Here's how the part is built. I have some questions about the finished solid (model axes, mm). A direction names the side the tool comes from. Round coordinates to 2 decimals unless told otherwise and drop trailing zeros. Write each loop counter-clockwise with the first axis right and the second up, starting at its lowest first coordinate (ties: lowest second). Pieces come first, ordered by that corner, then holes. Notation, with made-up numbers: (31, -24.75) - (66, -24.75) arc R21 ccw to (66, -20.75) - close; hole circle Ø9 at (44.5, 87). An arc over 180 degrees is marked (long way). Use one line per item in the form item = value. Start each with the question number.
1. I want a section at A-A, the plane x = 60. List the corners of the cut face in (y, z) for me.
2. I want a section at C-C, the plane y = 6. List the corners of the cut face in (x, z) for me.
3. I want a section at D-D, the plane x = 35. List the corners of the cut face in (y, z) for me.
4. I want a section at B-B, the plane z = 2. List the corners of the cut face in (x, y) for me.
5. Will these pins go through, and if not, where does the flat tip stop? pin 1 (6.5 mm diameter, centred on x = 6, y = 10, fed in from -Z); pin 2 (10 mm diameter, centred on x = 33, y = 7, fed in from -Z); pin 3 (1.5 mm diameter, centred on y = 3.5, z = 3.5, fed in from +X); pin 4 (2 mm diameter, centred on x = 62.5, z = 3.5, fed in from -Y).
6. If I drill on line 1 along X through (y, z) = (6, 2.25); line 2 along Y through (x, z) = (35, 0.35); line 3 along X through (y, z) = (11.5, 0.6), over which ranges is the centre line in solid material (lowest first)?
7. Which directions (+Z, -Z, +X, -X, +Y, -Y) give clear straight access to the entire face, cutting with the end or side of a thin tool? Please do faces 4 (the flat face through (37, 11, 1)), 5 (the cylindrical face through (35, -4, 2)), 6 (the flat face through (17, 0, 2)), 7 (the flat face through (35, 13, 4)), 8 (the flat face through (53, 0, 2)).
8. We'd pull the mould along Y, two halves only. Please class faces 1 (the cylindrical face through (67.9, 14, 2)), 2 (the cylindrical face through (57.4, 7.6, 2)), 3 (the flat face through (35, 15, 0)): +Y half, -Y half, draft (parallel to the pull), parting line (faces both ways), or undercut.
```python
from build123d import *

# Parameters (mm, degrees)
SKETCH_R     = 2.1
SKETCH_R_2   = 5
SKETCH_R_3   = 2.6
PAD_DEPTH    = 4
FILLET_R     = 7
FILLET001_R  = 7
SKETCH001_R  = 7.75
POCKET_DEPTH = 1


with BuildPart() as part:
    # Sketch → Pad (new body)
    with BuildSketch(Plane.XY):
        with BuildLine():
            Line((0, 0), (27, 0))
            ThreePointArc((27, 0), (35, -4), (43, 0))
            Line((43, 0), (70, 0))
            Line((70, 0), (70, 16))
            Line((70, 16), (0, 16))
            Line((0, 16), (0, 0))
        make_face()
        with Locations((6, 10)):
            Circle(SKETCH_R, mode=Mode.SUBTRACT)
        with Locations((35, 6)):
            Circle(SKETCH_R_2, mode=Mode.SUBTRACT)
        with Locations((60, 7.5)):
            Circle(SKETCH_R_3, mode=Mode.SUBTRACT)
    extrude(amount=PAD_DEPTH)

    # Fillet
    fillet_edges = [part.edges().sort_by_distance(p)[0] for p in [
        (70, 0, 2),
        (70, 16, 2),
    ]]
    fillet(fillet_edges, radius=FILLET_R)

    # Fillet001
    fillet001_edges = [part.edges().sort_by_distance(p)[0] for p in [
        (0, 0, 2),
        (0, 16, 2),
    ]]
    fillet(fillet001_edges, radius=FILLET001_R)

    # Sketch001 (on Face1 of Fillet001) → Pocket (cut)
    with BuildSketch(Plane(origin=(0, 0, 0), x_dir=(1, 0, 0), z_dir=(0, 0, -1))):
        with Locations((35, -6)):
            Circle(SKETCH001_R)
    extrude(amount=-POCKET_DEPTH, mode=Mode.SUBTRACT)


solid = part.part
```
Model answer:
q1.outline = (0, 0) - (4.9, 0) - (4.9, 4) - (0, 4) - close; (10.1, 0) - (16, 0) - (16, 4) - (10.1, 4) - close
q2.outline = (0.07, 0) - (27.25, 0) - (27.25, 1) - (30, 1) - (30, 4) - (0.07, 4) - close; (40, 1) - (42.75, 1) - (42.75, 0) - (57.88, 0) - (57.88, 4) - (40, 4) - close; (62.12, 0) - (69.93, 0) - (69.93, 4) - (62.12, 4) - close
q3.outline = (-4, 0) - (-1.75, 0) - (-1.75, 1) - (1, 1) - (1, 4) - (-4, 4) - close; (11, 1) - (13.75, 1) - (13.75, 0) - (16, 0) - (16, 4) - (11, 4) - close
q4.outline = (0, 7) arc R7 ccw to (7, 0) - (27, 0) arc R10 ccw to (43, 0) - (63, 0) arc R7 ccw to (70, 7) - (70, 9) arc R7 ccw to (63, 16) - (7, 16) arc R7 ccw to (0, 9) - close; hole circle Ø4.2 at (6, 10); hole circle Ø10 at (35, 6); hole circle Ø5.2 at (60, 7.5)
q5.pin_1 = 0
q5.pin_2 = 1
q5.pin_3 = 69.44
q5.pin_4 = 0
q6.line_1 = 0.07 to 30, 40 to 57.88, 62.12 to 69.93
q6.line_2 = -4 to -1.75, 13.75 to 16
q6.line_3 = 0.46 to 4.53, 7.47 to 29.54, 40.46 to 69.54
q7.face_4 = -Z
q7.face_5 = +Z, -Z, -Y
q7.face_6 = +Z, -Z, -X, -Y
q7.face_7 = +Z, +X, -X, +Y, -Y
q7.face_8 = +Z, -Z, +X, -Y
q8.face_1 = +Y half
q8.face_2 = undercut
q8.face_3 = draft
